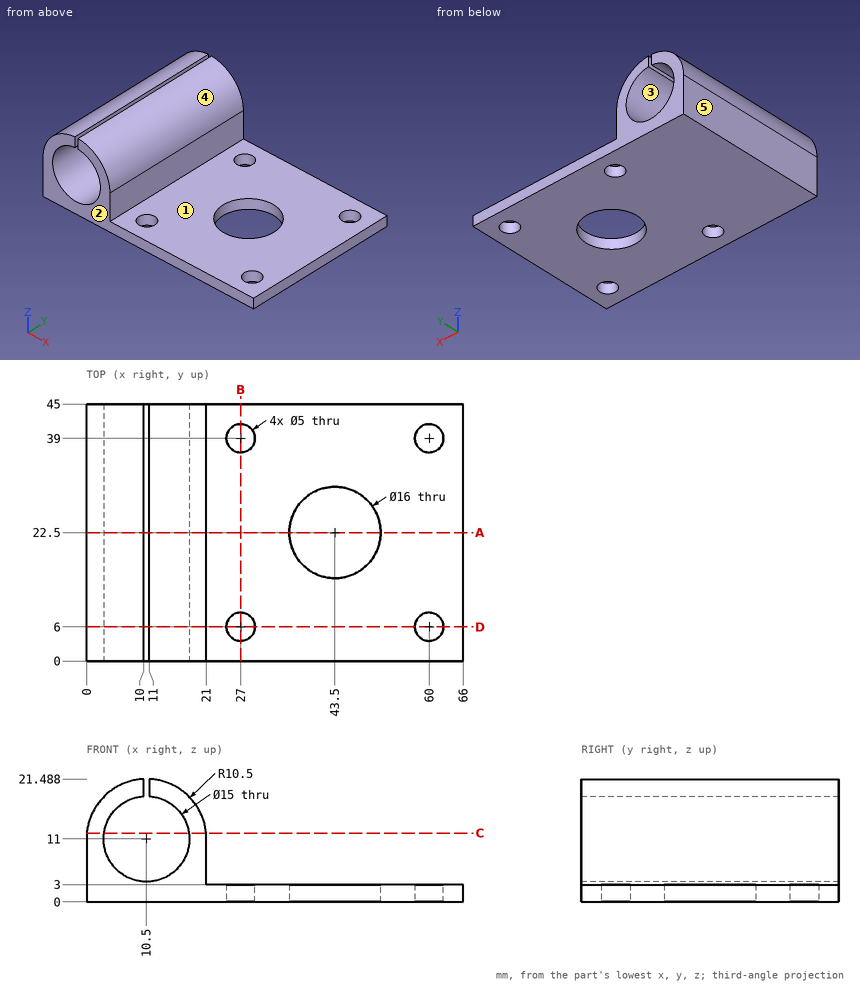
The drawing under review shows one solid part. Ordinate dimensions are in mm from its lowest x, y, z. A direction names the side the tool comes from. Round coordinates to 2 decimals unless told otherwise and drop trailing zeros. Loops run counter-clockwise (first coordinate to the right, second up) from the corner with the lowest first, then second, coordinate; pieces in that order, holes last. Notation, with made-up numbers: (67.5, 81) -> (79.5, 81) arc R28 cw to (79.5, 100) -> close; hole circle Ø1 at (33, 59). An arc over 180 degrees is marked (long way). Answer in a Markdown table with one row per item.
1) Consider section A-A, the plane y = 22.5. Write out the cut boundary in (x, z), plus the area to 3 significant figures.
Taken from the geometry:
| item | result |
|---|---|
| outline | (0, 0) -> (35.5, 0) -> (35.5, 3) -> (21, 3) -> (21, 11) arc R10.5 ccw to (11, 21.49) -> (11, 18.48) arc R7.5 cw (long way) to (10, 18.48) -> (10, 21.49) arc R10.5 ccw to (0, 11) -> close; (51.5, 0) -> (66, 0) -> (66, 3) -> (51.5, 3) -> close |
| area | 311 mm² |
2) Consider section D-D, the plane y = 6. Write out the cut boundary in (x, z).
Taken from the geometry:
| item | result |
|---|---|
| outline | (0, 0) -> (24.5, 0) -> (24.5, 3) -> (21, 3) -> (21, 11) arc R10.5 ccw to (11, 21.49) -> (11, 18.48) arc R7.5 cw (long way) to (10, 18.48) -> (10, 21.49) arc R10.5 ccw to (0, 11) -> close; (29.5, 0) -> (57.5, 0) -> (57.5, 3) -> (29.5, 3) -> close; (62.5, 0) -> (66, 0) -> (66, 3) -> (62.5, 3) -> close |
3) Wall thickness on line 1 along X through (y, z) = (6, 2.2); line 2 along Y through (x, z) = (60, 0.8); line 3 along X through (y, z) = (35, 10.5): over which ranges is each line inside the solid? List them lowest first.
Taken from the geometry:
| item | result |
|---|---|
| line 1 | x = 0 to 24.5, 29.5 to 57.5, 62.5 to 66 |
| line 2 | y = 0 to 3.5, 8.5 to 36.5, 41.5 to 45 |
| line 3 | x = 0 to 3.02, 17.98 to 21 |
4) Consider section C-C, the plane z = 12. Write out the cut boundary in (x, y).
Taken from the geometry:
| item | result |
|---|---|
| outline | (0.05, 0) -> (3.07, 0) -> (3.07, 45) -> (0.05, 45) -> close; (17.93, 0) -> (20.95, 0) -> (20.95, 45) -> (17.93, 45) -> close |
5) Draft analysis for pull direction X (two halves, no side actions). For the marked faces 3, 4 and 5, state which applies: pulls with the +X half, pulls with the -X half, needs draft (parallel to the pull), parting line crosses it, or undercut.
Taken from the geometry:
| item | result |
|---|---|
| face 3 | undercut |
| face 4 | pulls with the +X half |
| face 5 | pulls with the -X half |
6) For pin 1 Ø1.5 at (y, z) = (20, 20.5) entering from -X; pin 2 Ø6 at (y, z) = (10, 13.5) entering from +X; pin 3 Ø2.5 at (y, z) = (33.5, 20) entering from +X, all flat-tipped, find the tip position at first contact; note any pin that passes through.
Taken from the geometry:
| item | result |
|---|---|
| pin 1 | stops at x = 4.7 |
| pin 2 | stops at x = 21 |
| pin 3 | stops at x = 17.58 |
7) Tool access review of the marked faces 1 and 2: name each direction out of +Z, -Z, +X, -X, +Y, -Y from which nothing blocks a thin tool from reaching the whole face with its end or side.
Taken from the geometry:
| item | result |
|---|---|
| face 1 | +Z, +X, +Y, -Y |
| face 2 | +Z, -Z, +X, -X, -Y |
8) Consider section B-B, the plane x = 27. Write out the cut boundary in (y, z).
Taken from the geometry:
| item | result |
|---|---|
| outline | (0, 0) -> (3.5, 0) -> (3.5, 3) -> (0, 3) -> close; (8.5, 0) -> (36.5, 0) -> (36.5, 3) -> (8.5, 3) -> close; (41.5, 0) -> (45, 0) -> (45, 3) -> (41.5, 3) -> close |
